Geometry: see drawing. Coordinates: mm, zero at the bounding-box minimum. A direction names the side the tool comes from. Round coordinates to 2 decimals unless told otherwise and drop trailing zeros. Order: outer loops, then holes, each group sorted by start corner. A loop starts at its lowest first (then second) coordinate and runs counter-clockwise, first axis right, second up. Notation, with made-up numbers: (-20, -7) -> (3, -7) arc R12 cw to (3, 1) -> close; hole circle Ø3 at (40.5, 69). An arc over 180 degrees is marked (long way). Answer as CSV lines item,"result". Start each with the question number.
(1) Pull-direction query (Y, two-part tool) for the marked faces 6, 7 and 8; classes: +Y half, -Y half, draft (parallel to the pull), parting line (faces both ways), or undercut.
(2) Section query A-A (z = 16). Output: boundary loops of the cut face in (x, y), plus the area to 3 significant figures.
(3) Line query: line 1 along X through (y, z) = (4.25, 16.25); line 2 along Z through (x, y) = (11.25, 4.5); line 3 along Z through (x, y) = (12.25, 10.25). Output: solid intervals per line, ascending. Write a range as from..to.
(4) Section query C-C (x = 7.75). Output: boundary loops of the cut face in (y, z).
(5) Contact query for flat-ended pins moving along their axis: P1, Ø5, axis at x = 3.5, z = 7.5, coming from the -Y side; P2, Ø2.5, axis at x = 9, z = 16, coming from the -Y side; P3, Ø5.5, axis at x = 10, y = 7, coming from the -Z side; P4, Ø2, axis at x = 1.5, y = 4.5, coming from the -Z side. Output: stop coordinate, or through.
(6) Set-up query: the marked faces 1, 2, 3, 4 and 5. Return all of +Z, -Z, +X, -X, +Y, -Y with unobstructed straight access to the full face (end or side cutting, diameter ignored); none if empty.
(7) Section query D-D (y = 3.5). Output: boundary loops of the cut face in (x, z), plus the area to 3 significant figures.
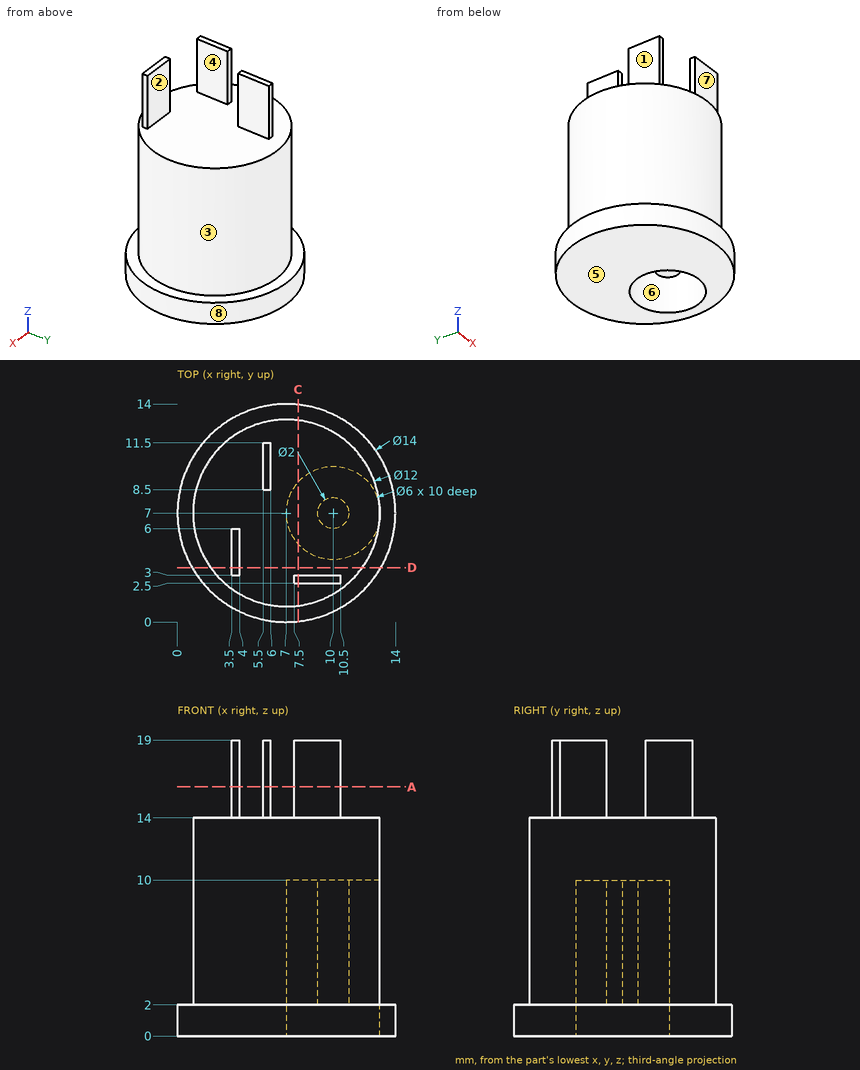
Answer block:
1,face 6,"undercut"
1,face 7,"-Y half"
1,face 8,"parting line"
2,outline,"(3.5, 3) -> (4, 3) -> (4, 6) -> (3.5, 6) -> close; (5.5, 8.5) -> (6, 8.5) -> (6, 11.5) -> (5.5, 11.5) -> close; (7.5, 2.5) -> (10.5, 2.5) -> (10.5, 3) -> (7.5, 3) -> close"
2,area,"4.50 mm2"
3,line 1,"3.5..4"
3,line 2,"10..14"
3,line 3,"0..2"
4,outline,"(0.04, 0) -> (5.02, 0) -> (5.02, 10) -> (8.98, 10) -> (8.98, 0) -> (13.96, 0) -> (13.96, 2) -> (12.95, 2) -> (12.95, 14) -> (3, 14) -> (3, 19) -> (2.5, 19) -> (2.5, 14) -> (1.05, 14) -> (1.05, 2) -> (0.04, 2) -> close"
5,P1,"y = 1.08"
5,P2,"y = 2.5"
5,P3,"z = 2"
5,P4,"z = 0"
6,face 1,"+Z, -X, +Y, -Y"
6,face 2,"+Z, +X, +Y"
6,face 3,"+Z"
6,face 4,"+Z, +X, +Y, -Y"
6,face 5,"-Z, +X, -X, +Y, -Y"
7,outline,"(0.94, 0) -> (13.06, 0) -> (13.06, 2) -> (11.87, 2) -> (11.87, 14) -> (4, 14) -> (4, 19) -> (3.5, 19) -> (3.5, 14) -> (2.13, 14) -> (2.13, 2) -> (0.94, 2) -> close"
7,area,"144 mm2"
